The model under review builds one solid part; all positions refer to its coordinate system, in mm. Face numbers are marked on the shaded views. A direction names the side the tool comes from. Round coordinates to 2 decimals unless told otherwise and drop trailing zeros. Order: outer loops, then holes, each group sorted by start corner. A loop starts at its lowest first (then second) coordinate and runs counter-clockwise, first axis right, second up.
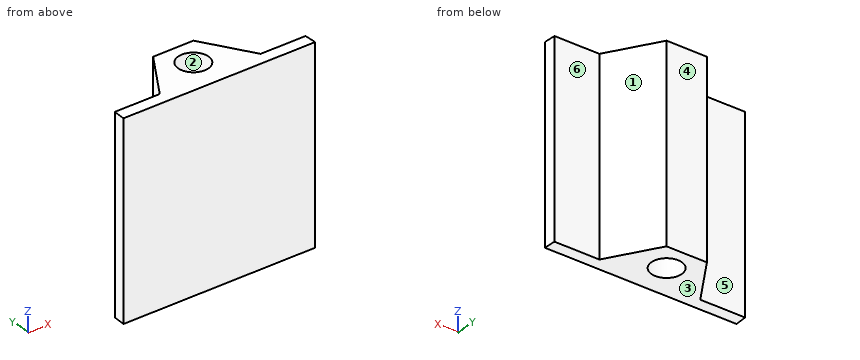
```python
from build123d import *

# Parameters (mm, degrees)
F1_DEPTH = 25.4
F2_R     = 4
F3_DEPTH = 25.4


with BuildPart() as f1:
    # F0 (on Top) → F1 (new body, symmetric)
    with BuildSketch(Plane.XY):
        Polygon((-25.4, 0), (0, 0), (25.4, 0), (25.266184, 3.175), (0, 3.175), (-25.266184, 3.175), align=None)
    extrude(amount=F1_DEPTH, both=True)

    # F2 (on Top) → F3 (join, symmetric)
    with BuildSketch(Plane.XY):
        Polygon((-5.34885, 16), (-15.349967, 0), (15.349967, 0), (5.34885, 16), (0, 16), align=None)
        with Locations((0, 9.023245)):
            Circle(F2_R, mode=Mode.SUBTRACT)
    extrude(amount=F3_DEPTH, both=True)


solid = f1.part
```
(1) Consider section C-C (z = 17). Write out the cut boundary in (x, y) (3 decimals).
Data:
outline: (-25.4, 0) - (25.4, 0) - (25.266, 3.175) - (13.365, 3.175) - (5.349, 16) - (-5.349, 16) - (-13.365, 3.175) - (-25.266, 3.175) - close; hole circle Ø8 at (0, 9.023)
(2) Draft analysis for pull direction Y (two halves, no side actions). For the marked faces 1, 2 and 3, state which applies: pulls with the +Y half, pulls with the -Y half, needs draft (parallel to the pull), parting line crosses it, or undercut.
Data:
face 1: pulls with the +Y half
face 2: undercut
face 3: needs draft
(3) Consider section B-B (x = 0). Write out the cut boundary in (y, z).
Data:
outline: (0, -25.4) - (5.02, -25.4) - (5.02, 25.4) - (0, 25.4) - close; (13.02, -25.4) - (16, -25.4) - (16, 25.4) - (13.02, 25.4) - close
(4) For the marked faces 4, 5 and 6, list the 3-axis set-ups (+Z, -Z, +X, -X, +Y, -Y) from which the entire face can be reached by the end or side of a thin tool; tool diameter is ignored.
Data:
face 4: +Z, -Z, +X, -X, +Y
face 5: +Z, -Z, -X, +Y
face 6: +Z, -Z, +X, +Y
(5) Consider section A-A (y = 7.25). Write out the cut boundary in (x, z), and give its area (3 significant figures).
Data:
outline: (-10.82, -25.4) - (-3.59, -25.4) - (-3.59, 25.4) - (-10.82, 25.4) - close; (3.59, -25.4) - (10.82, -25.4) - (10.82, 25.4) - (3.59, 25.4) - close
area: 735 mm2
(6) Insertion check: pin 1 (6 mm diameter, centred on y = 8.5, z = 2, fed in from -X); pin 2 (3 mm diameter, centred on y = 8.5, z = -2.5, fed in from -X); pin 3 (9.5 mm diameter, centred on x = -19.5, z = 2, fed in from +Y) (3 decimals); pin 4 (8 mm diameter, centred on x = -16, y = 11, fed in from -Z). Each pin has a flat end and moves straight along its axis. Give the tip position at first contact, or say it passes through.
Data:
pin 1: stops at x = -11.91
pin 2: stops at x = -10.97
pin 3: stops at y = 3.175
pin 4: passes through
(7) Consider section D-D (x = 16). Write out the cut boundary in (y, z) (3 decimals), and give its area (3 significant figures).
Data:
outline: (0, -25.4) - (3.175, -25.4) - (3.175, 25.4) - (0, 25.4) - close
area: 161 mm2
(8) To check wall thickness, follow probe 1 along Y at (x, z) = (0, -16.5); probe 2 along Y at (x, z) = (7, 16); probe 3 along Y at (x, z) = (19, 11.5) (3 decimals). State the ranges of each line that lie inside material, in increasing order.
Data:
probe 1: y = 0 to 5.02, 13.02 to 16
probe 2: y = 0 to 13.36
probe 3: y = 0 to 3.175
